Part model, mm, in its own coordinate system. Round coordinates to 2 decimals unless told otherwise and drop trailing zeros. Loops run counter-clockwise (first coordinate to the right, second up) from the corner with the lowest first, then second, coordinate; pieces in that order, holes last.
(1) Probe probe 1 along Y at (x, z) = (-37.5, 3.2); probe 2 along X at (y, z) = (37, 2.05); probe 3 along X at (y, z) = (34, 0.9). List the from-to ranges inside material, lowest first.
(2) Cut at D-D on z = 2.05. List the corners of the cut face in (x, y).
(3) Cut at A-A on y = -37.5. List the corners of the cut face in (x, z).
(4) Flat gauge pins, fed straight in: pin 1 (1 mm diameter, centred on x = -10, y = 18.5, fed in from -Z); pin 2 (2 mm diameter, centred on x = -11, z = 2.5, fed in from +Y). Where does each tip first touch, or does it go through?
(5) Cut at B-B on y = 37.5. List the corners of the cut face in (x, z).
from build123d import *

# Parameters (mm, degrees)
SKETCH1_W           = 100
SKETCH1_H           = 100
BOSS_EXTRUDE1_DEPTH = 4
SKETCH2_R           = 2.6
CUT_EXTRUDE1_DEPTH  = 4
FILLET1_R           = 5
SKETCH3_W           = 55
SKETCH3_H           = 25
CUT_EXTRUDE2_DEPTH  = 4


with BuildPart() as part:
    # Sketch1 → Boss-Extrude1 (new body)
    with BuildSketch(Plane.XY):
        Rectangle(SKETCH1_W, SKETCH1_H)
    extrude(amount=BOSS_EXTRUDE1_DEPTH)

    # Sketch2 → Cut-Extrude1 (cut)
    with BuildSketch(Plane.XY.offset(4)):
        with Locations((-37.5, 37.5)):
            Circle(SKETCH2_R)
        with Locations((-37.5, -37.5)):
            Circle(SKETCH2_R)
        with Locations((37.5, -37.5)):
            Circle(SKETCH2_R)
        with Locations((37.5, 37.5)):
            Circle(SKETCH2_R)
    extrude(amount=-CUT_EXTRUDE1_DEPTH, mode=Mode.SUBTRACT)

    # Fillet1
    fillet1_edges = [part.edges().sort_by_distance(p)[0] for p in [
        (-50, 50, 2),
        (50, 50, 2),
        (50, -50, 2),
        (-50, -50, 2),
    ]]
    fillet(fillet1_edges, radius=FILLET1_R)

    # Sketch3 → Cut-Extrude2 (cut)
    with BuildSketch(Plane(origin=(0, 0, 0), x_dir=(-1, 0, 0), z_dir=(0, 0, -1))):
        with Locations((0, 43.482027076)):
            Rectangle(SKETCH3_W, SKETCH3_H)
    extrude(amount=-CUT_EXTRUDE2_DEPTH, mode=Mode.SUBTRACT)


solid = part.part
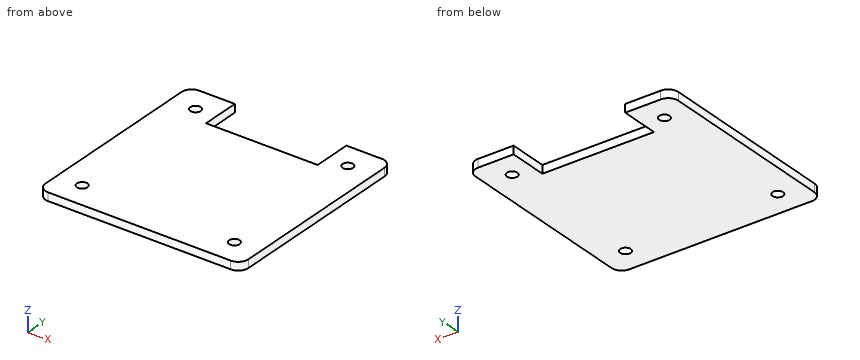
Final values:
1. probe 1: y = -50 to -40.1, -34.9 to 34.9, 40.1 to 50
1. probe 2: x = -50 to -40.05, -34.95 to -27.5, 27.5 to 34.95, 40.05 to 50
1. probe 3: x = -50 to -27.5, 27.5 to 50
2. outline: (-50, -45) arc R5 ccw to (-45, -50) - (45, -50) arc R5 ccw to (50, -45) - (50, 45) arc R5 ccw to (45, 50) - (27.5, 50) - (27.5, 30.98) - (-27.5, 30.98) - (-27.5, 50) - (-45, 50) arc R5 ccw to (-50, 45) - close; hole circle Ø5.2 at (-37.5, -37.5); hole circle Ø5.2 at (-37.5, 37.5); hole circle Ø5.2 at (37.5, -37.5); hole circle Ø5.2 at (37.5, 37.5)
3. outline: (-50, 0) - (-40.1, 0) - (-40.1, 4) - (-50, 4) - close; (-34.9, 0) - (34.9, 0) - (34.9, 4) - (-34.9, 4) - close; (40.1, 0) - (50, 0) - (50, 4) - (40.1, 4) - close
4. pin 1: stops at z = 0
4. pin 2: stops at y = 30.98
5. outline: (-50, 0) - (-40.1, 0) - (-40.1, 4) - (-50, 4) - close; (-34.9, 0) - (-27.5, 0) - (-27.5, 4) - (-34.9, 4) - close; (27.5, 0) - (34.9, 0) - (34.9, 4) - (27.5, 4) - close; (40.1, 0) - (50, 0) - (50, 4) - (40.1, 4) - close
